For this review, take the finished solid that the model builds, in its own axes (mm). Coordinates: 2 decimals unless noted, no trailing zeros. Order: outer loops, then holes, each group sorted by start corner. A loop starts at its lowest first (then second) coordinate and runs counter-clockwise, first axis right, second up. Notation, with made-up numbers: M 8.5,22 L 35.5,22 A7 ccw 35.5,27 Z; hole C -30,39.25 d6. An arc over 180 degrees is marked long. Use one line per item in the form item = value. Start each with the question number.
```python
from build123d import *

# Parameters (mm, degrees)
F0_W     = 126.9580200315
F0_H     = 84.6386812627
F1_DEPTH = 127
F2_SIZE2 = 36.2749593712
F2_SIZE  = 25.4
F3_R     = 1.27


with BuildPart() as f1:
    # F0 (on Front) → F1 (new body, symmetric)
    with BuildSketch(Plane.XZ):
        with Locations((0.826548785, 2.1490287036)):
            Rectangle(F0_W, F0_H)
    extrude(amount=F1_DEPTH, both=True)

    # F2
    f2_edges = [f1.edges().sort_by_distance(p)[0] for p in [
        (0.826549, -127, 44.468369),
    ]]
    f2_side = f1.faces().sort_by_distance((0.826549, 0, 44.468369))[0]
    chamfer(f2_edges, length=F2_SIZE, length2=F2_SIZE2, reference=f2_side)

    # F3
    f3_edges = [f1.edges().sort_by_distance(p)[0] for p in [
        (0.826549, 127, 44.468369),
        (-62.652461, 127, 2.149029),
        (0.826549, 127, -40.170312),
        (64.305559, 127, 2.149029),
        (-62.652461, -127, -15.988451),
        (0.826549, -127, 8.19341),
        (0.826549, -127, -40.170312),
        (64.305559, -127, -15.988451),
    ]]
    fillet(f3_edges, radius=F3_R)


solid = f1.part
```
1. For pin 1 Ø5 at (x, z) = (40, 29) entering from -Y, flat-tipped, find the tip position at first contact; note if it passes through.
2. Consider section A-A, the plane x = 0. Write out the cut boundary in (y, z), plus the area to 3 significant figures.
3. To check wall thickness, follow line 1 (Y direction, x = 9.5, z = 8); line 2 (Y direction, x = 54, z = 13.5). State the ranges of each line that lie inside material, in increasing order.
Answers follow:
q1.pin_1 = -114.18
q2.outline = M -127,-38.9 A1.27 ccw -125.73,-40.17 L 125.73,-40.17 A1.27 ccw 127,-38.9 L 127,43.2 A1.27 ccw 125.73,44.47 L -101.6,44.47 L -126.77,8.52 A1.27 ccw -127,7.79 Z
q2.area = 21,000 mm²
q3.line_1 = -126.98 to 127
q3.line_2 = -123.28 to 127
